from build123d import *

# Parameters (mm, degrees)
SKETCH1_W           = 45
SKETCH1_H           = 20
BOSS_EXTRUDE1_DEPTH = 1
SKETCH2_R           = 7.5
SKETCH2_R_2         = 6
BOSS_EXTRUDE2_DEPTH = 12
BOSS_EXTRUDE3_DEPTH = 2
BOSS_EXTRUDE4_START = -0.5
SKETCH4_R           = 6
BOSS_EXTRUDE4_DEPTH = 0.1
SKETCH9_W           = 0.5
SKETCH9_H           = 0.5
SKETCH9_2_W         = 0.5
SKETCH9_2_H         = 0.5
BOSS_EXTRUDE7_DEPTH = 1.5
LPATTERN5_COUNT     = 4
LPATTERN5_PITCH     = 2.5
BOSS_EXTRUDE6_DEPTH = 2.5
SKETCH12_R          = 1
CUT_EXTRUDE4_DEPTH  = 1.5


with BuildPart() as part:
    # Sketch1 → Boss-Extrude1 (new body)
    with BuildSketch(Plane(origin=(0, 0, 0), x_dir=(1, 0, 0), z_dir=(0, 1, 0))):
        Rectangle(SKETCH1_W, SKETCH1_H)
    extrude(amount=BOSS_EXTRUDE1_DEPTH)

    # Sketch2 → Boss-Extrude2 (add)
    # profile 1 of 2: a face of its own
    with BuildSketch(Plane(origin=(0, 1, 0), x_dir=(1, 0, 0), z_dir=(0, 1, 0))):
        with Locations(Location((-12.5, 0, 0), (0, 0, 270))):
            Circle(SKETCH2_R)
        with Locations(Location((-12.5, 0, 0), (0, 0, 270))):
            Circle(SKETCH2_R_2, mode=Mode.SUBTRACT)
    # profile 2 of 2: a face of its own
    with BuildSketch(Plane(origin=(0, 1, 0), x_dir=(1, 0, 0), z_dir=(0, 1, 0))):
        with Locations(Location((12.5, 0, 0), (0, 0, 90))):
            Circle(SKETCH2_R)
        with Locations(Location((12.5, 0, 0), (0, 0, 90))):
            Circle(SKETCH2_R_2, mode=Mode.SUBTRACT)
    extrude(amount=BOSS_EXTRUDE2_DEPTH)

    # Sketch3 → Boss-Extrude3 (add)
    with BuildSketch(Plane(origin=(0, 1, 0), x_dir=(1, 0, 0), z_dir=(0, 1, 0))):
        with BuildLine():
            Line((-3, 9), (3, 9))
            ThreePointArc((3, 9), (4.75, 7.25), (3, 5.5))
            Line((3, 5.5), (-3, 5.5))
            ThreePointArc((-3, 5.5), (-4.75, 7.25), (-3, 9))
        make_face()
    extrude(amount=BOSS_EXTRUDE3_DEPTH)

    # Sketch4 → Boss-Extrude4 (add)
    with BuildSketch(Plane(origin=(0, 13, 0), x_dir=(1, 0, 0), z_dir=(0, 1, 0)).offset(BOSS_EXTRUDE4_START)):
        with Locations(Location((-12.5, 0, 0), (0, 0, 270))):
            Circle(SKETCH4_R)
        with Locations(Location((12.5, 0, 0), (0, 0, 90))):
            Circle(SKETCH4_R)
    extrude(amount=BOSS_EXTRUDE4_DEPTH)

    # Sweep1: sweep along a path in Sketch8
    with BuildLine(Plane(origin=(3.75, 0, 0), x_dir=(0, 0, -1), z_dir=(1, 0, 0))) as sweep1_path:
        Line((-8.75, 0), (-8.75, -3))
        ThreePointArc((-8.75, -3), (-9.042893219, -3.707106781), (-9.75, -4))
        Line((-9.75, -4), (-16.25, -4))
    # Sketch9 → Sweep1 (sweep)
    with BuildSketch(Plane.XZ):
        with Locations((3.75, 8.75)):
            Rectangle(SKETCH9_W, SKETCH9_H)
    sweep1 = sweep(path=sweep1_path.line)

    # Sketch9<2> → Boss-Extrude7 (add)
    with BuildSketch(Plane.XZ):
        with Locations((3.75, 8.75)):
            Rectangle(SKETCH9_2_W, SKETCH9_2_H)
    boss_extrude7 = extrude(amount=-BOSS_EXTRUDE7_DEPTH)

    # LPattern5: Sweep1, Boss-Extrude7 ×4
    with Locations(*[(-i * LPATTERN5_PITCH, 0, 0) for i in range(1, LPATTERN5_COUNT)]):
        add(sweep1)
        add(boss_extrude7)

    # Sketch11 → Boss-Extrude6 (add)
    with BuildSketch(Plane.XZ):
        Polygon((3, 7.5), (4.5, 7.5), (5, 8), (5, 9.5), (4.5, 10), (3, 10), (2.5, 9.5), (2, 10), (0.5, 10), (0, 9.5), (-0.5, 10), (-2, 10), (-2.5, 9.5), (-3, 10), (-4.5, 10), (-5, 9.5), (-5, 8), (-4.5, 7.5), (-3, 7.5), (-2.5, 8), (-2, 7.5), (-0.5, 7.5), (0, 8), (0.5, 7.5), (2, 7.5), (2.5, 8), align=None)
    extrude(amount=BOSS_EXTRUDE6_DEPTH)

    # Sketch12 → Cut-Extrude4 (cut)
    with BuildSketch(Plane.XZ):
        with Locations(Location((-21, 8.5, 0), (0, 0, 270))):
            Circle(SKETCH12_R)
        with Locations(Location((-21, -8.5, 0), (0, 0, 90))):
            Circle(SKETCH12_R)
        with Locations(Location((21, -8.5, 0), (0, 0, 270))):
            Circle(SKETCH12_R)
        with Locations(Location((21, 8.5, 0), (0, 0, 90))):
            Circle(SKETCH12_R)
    extrude(amount=-CUT_EXTRUDE4_DEPTH, mode=Mode.SUBTRACT)


solid = part.part
Could you check a few things on this model? Use its own coordinates, in mm. A direction names the side the tool comes from. Coordinates: 2 decimals unless noted, no trailing zeros. Loops run counter-clockwise (first coordinate to the right, second up) from the corner with the lowest first, then second, coordinate; pieces in that order, holes last. Notation, with made-up numbers: (9, -11) -> (59, -11) arc R25 cw to (59, 9) -> close; hole circle Ø7 at (32.5, 77). An arc over 180 degrees is marked (long way). Answer in a Markdown table with one row per item.
(1) Imagine slicing it at B-B (x = 12.5). List the corners of the cut face in (y, z) for me.
Results found:
| item | result |
|---|---|
| outline | (0, -10) -> (1, -10) -> (1, -7.5) -> (13, -7.5) -> (13, -6) -> (12.6, -6) -> (12.6, 6) -> (13, 6) -> (13, 7.5) -> (1, 7.5) -> (1, 10) -> (0, 10) -> close; hole (1, -6) -> (12.5, -6) -> (12.5, 6) -> (1, 6) -> close |
(2) Thinking about a two-plate mould opening in Z: for faces 6 (the face through (0, -2.5, 9)), 7 (the face through (12, 1, 0)), 8 (the face through (4, -1, 7.5)), which applies, released by +Z, released by -Z, zero draft, split by the parting line, or undercut?
Results found:
| item | result |
|---|---|
| face 6 | zero draft |
| face 7 | undercut |
| face 8 | released by -Z |
(3) Imagine slicing it at D-D (z = 0). List the corners of the cut face in (x, y) for me, plus the area to 3 significant figures.
Results found:
| item | result |
|---|---|
| outline | (-22.5, 0) -> (22.5, 0) -> (22.5, 1) -> (20, 1) -> (20, 13) -> (18.5, 13) -> (18.5, 12.6) -> (6.5, 12.6) -> (6.5, 13) -> (5, 13) -> (5, 1) -> (-5, 1) -> (-5, 13) -> (-6.5, 13) -> (-6.5, 12.6) -> (-18.5, 12.6) -> (-18.5, 13) -> (-20, 13) -> (-20, 1) -> (-22.5, 1) -> close; hole (-18.5, 1) -> (-6.5, 1) -> (-6.5, 12.5) -> (-18.5, 12.5) -> close; hole (6.5, 1) -> (18.5, 1) -> (18.5, 12.5) -> (6.5, 12.5) -> close |
| area | 119 mm^2 |
(4) Imagine slicing it at C-C (x = 21). List the corners of the cut face in (y, z) for me.
Results found:
| item | result |
|---|---|
| outline | (0, -10) -> (1, -10) -> (1, -9.5) -> (0, -9.5) -> close; (0, -7.5) -> (1, -7.5) -> (1, 7.5) -> (0, 7.5) -> close; (0, 9.5) -> (1, 9.5) -> (1, 10) -> (0, 10) -> close |
(5) For faces 1 (the face through (5, -1, 9)), 2 (the face through (-6.55, 6.67, -0.78)), 3 (the face through (3.5, -4, 12)), 4 (the face through (-6.55, 12.8, -0.78)), 5 (the face through (0, 2, -9)), which set-ups out of +Z, -Z, +X, -X, +Y, -Y let a thin tool reach every point of the face, with its end or its side?
Results found:
| item | result |
|---|---|
| face 1 | +Z, -Z, +X, -Y |
| face 2 | none |
| face 3 | +Z, -Z, -Y |
| face 4 | +Y |
| face 5 | -Z, +X, -X, +Y |
(6) Imagine slicing it at A-A (z = 14.5). List the corners of the cut face in (x, y) for me, plus the area to 3 significant figures.
Results found:
| item | result |
|---|---|
| outline | (-4, -4.25) -> (-3.5, -4.25) -> (-3.5, -3.75) -> (-4, -3.75) -> close; (-1.5, -4.25) -> (-1, -4.25) -> (-1, -3.75) -> (-1.5, -3.75) -> close; (1, -4.25) -> (1.5, -4.25) -> (1.5, -3.75) -> (1, -3.75) -> close; (3.5, -4.25) -> (4, -4.25) -> (4, -3.75) -> (3.5, -3.75) -> close |
| area | 1.00 mm^2 |
(7) If I drill on probe 1 along X at (y, z) = (0.8, -8.5); probe 2 along X at (y, z) = (12.95, 0); probe 3 along Z at (x, y) = (8.5, 0.5), over which ranges is the centre line in solid material (lowest first)?
Results found:
| item | result |
|---|---|
| probe 1 | x = -22.5 to -22, -20 to 20, 22 to 22.5 |
| probe 2 | x = -20 to -18.5, -6.5 to -5, 5 to 6.5, 18.5 to 20 |
| probe 3 | z = -10 to 10 |
(8) Will these pins go through, and if not, where does the flat tip stop? pin 1 Ø10 at (x, z) = (-15.5, 10) entering from +Y; pin 2 Ø3 at (x, y) = (5.5, 8) entering from +Z; pin 3 Ø2.5 at (x, z) = (-21, 8.5) entering from -Y; pin 4 Ø0.8 at (x, y) = (-1.5, -1.5) entering from -Z.
Results found:
| item | result |
|---|---|
| pin 1 | stops at y = 13 |
| pin 2 | stops at z = 5.1 |
| pin 3 | stops at y = 0 |
| pin 4 | stops at z = 7.5 |
